Autodesk Inventor part; units mm, degrees
ref_plane "YZ Plane" through (0, 0, 0) normal (1, 0, 0) x (0, 1, 0)
ref_plane "XZ Plane" through (0, 0, 0) normal (0, 1, 0) x (-1, 0, 0)
ref_plane "XY Plane" through (0, 0, 0) normal (0, 0, 1) x (1, 0, 0)
sketch "スケッチ1" plane through (0, 0, 0) normal (0, 1, 0) x (-1, 0, 0)
  line L0 (15.5, -10.75) -> (-15.5, -10.75)
  line L1 (-15.5, -10.75) -> (-15.5, 10.75)
  line L2 (-15.5, 10.75) -> (15.5, 10.75)
  line L3 (15.5, 10.75) -> (15.5, -10.75)
  line L4 (15.5, -10.75) -> (-15.5, 10.75)
  point P0 (0, 0)
  point P1 (0, 0)
  dimension "d0" = 31
  dimension "d1" = 21.5
extrude "押し出し1" add sketch "スケッチ1" along normal blind 10.5
fillet "フィレット1" radius 3 11 edges at (15.5, 10.5, 0) (0, 10.5, 10.75) (0, 0, 10.75) (15.5, 5.25, 10.75) (15.5, 0, 0) (15.5, 5.25, -10.75) (0, 10.5, -10.75) (-15.5, 10.5, 0) (-15.5, 5.25, -10.75) (-15.5, 0, 0) (0, 0, -10.75)
ref_plane "作業平面1" through (0, 3, -7.75) normal (1, 0, 0) x (0, 0, -1)
fillet "フィレット2" radius 3 3 edges at (-14.6213, 9.6213, 9.8713) (-14.6213, 0.8787, 9.8713) (-15.5, 5.25, 10.75)
properties part number "battery" material "LCP プラスチック"
Model file for the job. Use its own axes, mm. Round coordinates to 2 decimals unless told otherwise and drop trailing zeros. Write each loop counter-clockwise with the first axis right and the second up, starting at its lowest first coordinate (ties: lowest second). Pieces come first, ordered by that corner, then holes. Notation, with made-up numbers: M -19,28.25 L -1,28.25 A20 ccw -1,58.25 Z; hole C 66,-5 d11. An arc over 180 degrees is marked long. Put each result on its own line as item: value.
Item 1: Cut at B-B (x = 8). List the corners of the cut face in (y, z).
Responses:
outline: M 0,-7.75 A3 ccw 3,-10.75 L 7.5,-10.75 A3 ccw 10.5,-7.75 L 10.5,7.75 A3 ccw 7.5,10.75 L 3,10.75 A3 ccw 0,7.75 Z
Item 2: Cut at A-A (z = 2.25). List the corners of the cut face in (x, y).
Responses:
outline: M -15.5,3 A3 ccw -12.5,0 L 12.5,0 A3 ccw 15.5,3 L 15.5,7.5 A3 ccw 12.5,10.5 L -12.5,10.5 A3 ccw -15.5,7.5 Z
Item 3: Probe L1, parallel to X at y = 2.75, z = 3; L2, parallel to X at y = 7.5, z = 8.5; L3, parallel to Z at x = -13, y = 1.5. List the from-to ranges inside material, lowest first. Write a range as from..to.
Responses:
L1: -15.49..15.49
L2: -15.4..15.4
L3: -10.3..10.3
